Input: part model. Units: mm. Frame: model coordinates. A direction names the side the tool comes from. Give positions to 0.01 mm unless a question says otherwise; leave off trailing zeros. Order: outer loops, then holes, each group sorted by start corner. A loop starts at its lowest first (then second) coordinate and runs counter-clockwise, first axis right, second up. Notation, with made-up numbers: (-7.5, 79.5) - (6.5, 79.5) arc R27 ccw to (6.5, 104.5) - close; hole circle Ø7 at (25.25, 15.25). An arc over 180 degrees is marked (long way). Answer in a Markdown table with one row per item. Add a question column.
1. Ray query, line 1 (X direction, y = 1, z = -2.5); line 2 (X direction, y = 2, z = 2); line 3 (Y direction, x = 59.75, z = -2.25). Return the intervals inside material, ascending. Write a range as [from, to].
2. Section query D-D on y = 17. Return loops of the section in (x, z).
3. Section query A-A on y = 0. Return loops of the section in (x, z).
4. Access query for faces 1 (the face through (-69, 5, -7)), 2 (the face through (78.826, 6.007, -0.27)). Directions: +Z, -Z, +X, -X, +Y, -Y. A direction counts if a zero-diameter tool reaches every point of the face in a straight line with its end or side. Return the directions, or none.
5. Mould query, pull axis X, two halves, no side actions, for faces 3 (the face through (-79.73, 0.88, -0.27)), 4 (the face through (-1, 0, 0)), 5 (the face through (-1, -20, 5)). Classes: released by +X, released by -X, zero draft, split by the parting line, or undercut.
6. Contact query for flat-ended pins moving along their axis: pin 1 (12 mm diameter, centred on x = -59.75, y = 0, fed in from +Z); pin 2 (1 mm diameter, centred on y = -12, z = 2.5, fed in from -X). Output: stop coordinate, or through.
7. Section query C-C on x = -66. Return loops of the section in (y, z).
8. Section query B-B on z = 3.5. Return loops of the section in (x, y), and give its area (3 significant figures).
```python
from build123d import *

# Parameters (mm, degrees)
SCHIZZO1_W                   = 119.5
SCHIZZO1_H                   = 40
ESTRUSIONE_ESTRUSIONE1_DEPTH = 10
SCHIZZO2_R                   = 20
ESTRUSIONE_ESTRUSIONE2_DEPTH = 17
SCHIZZO3_R                   = 12.5
SCHIZZO3_R_2                 = 10
TAGLIO_ESTRUSIONE1_DEPTH     = 84.958695202


with BuildPart() as part:
    # Schizzo1 → Estrusione-Estrusione1 (new body)
    with BuildSketch(Plane.XY):
        Rectangle(SCHIZZO1_W, SCHIZZO1_H)
    extrude(amount=ESTRUSIONE_ESTRUSIONE1_DEPTH)

    # Schizzo2 → Estrusione-Estrusione2 (add)
    with BuildSketch(Plane.XY.offset(10)):
        with Locations((-59.75, 0)):
            Circle(SCHIZZO2_R)
        with Locations((59.75, 0)):
            Circle(SCHIZZO2_R)
    extrude(amount=-ESTRUSIONE_ESTRUSIONE2_DEPTH)

    # Schizzo3 → Taglio-Estrusione1 (cut, through all)
    with BuildSketch(Plane(origin=(0, 0, -7), x_dir=(-1, 0, 0), z_dir=(0, 0, -1))):
        with Locations((-59.75, 0)):
            Circle(SCHIZZO3_R)
        with Locations((59.75, 0)):
            Circle(SCHIZZO3_R_2)
    extrude(amount=-TAGLIO_ESTRUSIONE1_DEPTH, mode=Mode.SUBTRACT)


solid = part.part
```
Answer:
| question | item | result |
|---|---|---|
| 1 | line 1 | x = [-79.72, -69.7], [-49.8, -39.78], [39.78, 47.29], [72.21, 79.72] |
| 1 | line 2 | x = [-79.65, -69.55], [-49.95, 47.41], [72.09, 79.65] |
| 1 | line 3 | y = [-20, -12.5], [12.5, 20] |
| 2 | outline | (-70.29, -7) - (-49.21, -7) - (-49.21, 0) - (49.21, 0) - (49.21, -7) - (70.29, -7) - (70.29, 10) - (-70.29, 10) - close |
| 3 | outline | (-79.75, -7) - (-69.75, -7) - (-69.75, 10) - (-79.75, 10) - close; (-49.75, -7) - (-39.75, -7) - (-39.75, 0) - (39.75, 0) - (39.75, -7) - (47.25, -7) - (47.25, 10) - (-49.75, 10) - close; (72.25, -7) - (79.75, -7) - (79.75, 10) - (72.25, 10) - close |
| 4 | face 1 | -Z, +X, -X, +Y, -Y |
| 4 | face 2 | -Z |
| 5 | face 3 | undercut |
| 5 | face 4 | undercut |
| 5 | face 5 | zero draft |
| 6 | pin 1 | passes through |
| 6 | pin 2 | stops at x = -76.11 |
| 7 | outline | (-19, -7) - (-7.81, -7) - (-7.81, 10) - (-19, 10) - close; (7.81, -7) - (19, -7) - (19, 10) - (7.81, 10) - close |
| 8 | outline | (-59.75, -20) - (59.75, -20) arc R20 ccw to (59.75, 20) - (-59.75, 20) arc R20 ccw to start; hole circle Ø20 at (-59.75, 0); hole circle Ø25 at (59.75, 0) |
| 8 | area | 5,230 mm² |
